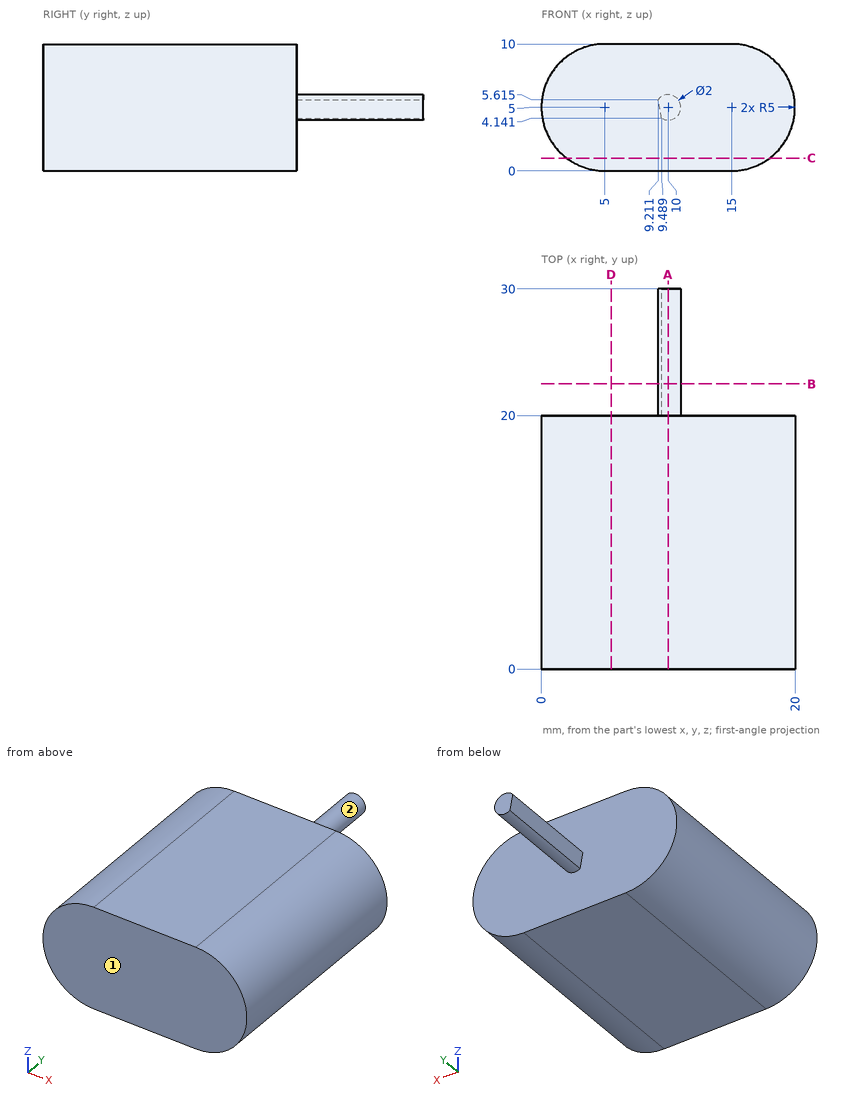
Job drawing, mm, ordinate dimensions from the low corner. One solid piece. A direction names the side the tool comes from. Round coordinates to 2 decimals unless told otherwise and drop trailing zeros. Write each loop counter-clockwise with the first axis right and the second up, starting at its lowest first coordinate (ties: lowest second). Pieces come first, ordered by that corner, then holes.
1) Drill centre lines: probe 1 along Y at (x, z) = (10, 8.5); probe 2 along Z at (x, y) = (10, 24); probe 3 along X at (y, z) = (25.25, 5.75). Where is each one in solid material? Low to high.
2) Band-saw the part on B-B, the plane y = 22.5. List the corners of the cut face in (x, z) (1 decimal).
3) Band-saw the part on D-D, the plane x = 5.5. List the corners of the cut face in (y, z).
4) Pin check, flat tips, straight feed: pin 1 (2 mm diameter, centred on x = 10.5, y = 21.5, fed in from -Z); pin 2 (1.5 mm diameter, centred on x = 5, z = 5.5, fed in from +Y). Stop position of each tip, or through.
5) 3-axis set-ups, long thin cutter, end or side, ignore diameter. For the marked faces 1 and 2: which of +Z, -Z, +X, -X, +Y, -Y reach the whole face in a straight line?
6) Band-saw the part on C-C, the plane z = 1. List the corners of the cut face in (x, y).
7) Band-saw the part on A-A, the plane x = 10. List the corners of the cut face in (y, z), and give its area (3 significant figures).
Ans:
1. probe 1: y = 0 to 20
1. probe 2: z = 4 to 6
1. probe 3: x = 9.34 to 10.66
2. outline: (9.2, 5.6) - (9.5, 4.1) arc R1 ccw (long way) to start
3. outline: (0, 0) - (20, 0) - (20, 10) - (0, 10) - close
4. pin 1: stops at z = 4
4. pin 2: stops at y = 20
5. face 1: +Z, -Z, +X, -X, -Y
5. face 2: +Y
6. outline: (2, 0) - (18, 0) - (18, 20) - (2, 20) - close
7. outline: (0, 0) - (20, 0) - (20, 4) - (30, 4) - (30, 6) - (20, 6) - (20, 10) - (0, 10) - close
7. area: 220 mm2
